from build123d import *

# Parameters (mm, degrees)
SKETCH1_W           = 14.393333334
SKETCH1_H           = 14.393333333
BOSS_EXTRUDE1_DEPTH = 16
FILLET1_R           = 1
SKETCH2_R           = 5.926666667
CUT_EXTRUDE1_DEPTH  = 0.2


with BuildPart() as part:
    # Sketch1 → Boss-Extrude1 (new body)
    with BuildSketch(Plane.XY):
        with Locations((-166.361835023, 44.90232352)):
            Rectangle(SKETCH1_W, SKETCH1_H)
    extrude(amount=BOSS_EXTRUDE1_DEPTH)

    # Fillet1
    fillet1_edges = [part.edges().sort_by_distance(p)[0] for p in [
        (-159.165168356, 37.705656853, 8),
        (-173.55850169, 37.705656853, 8),
        (-173.55850169, 52.098990186, 8),
        (-159.165168356, 52.098990186, 8),
    ]]
    fillet(fillet1_edges, radius=FILLET1_R)

    # Sketch2 → Cut-Extrude1 (cut)
    with BuildSketch(Plane.XY.offset(16)):
        with Locations((-166.361835023, 44.902323519)):
            Circle(SKETCH2_R)
    extrude(amount=-CUT_EXTRUDE1_DEPTH, mode=Mode.SUBTRACT)


solid = part.part
Geometry: final body of the model. Coordinates: model frame, mm. Round coordinates to 2 decimals unless told otherwise and drop trailing zeros.
Q1. Pin query (flat end, axial travel): P1, Ø2, axis at x = -166.5, y = 40.5, coming from the +Z side; P2, Ø4, axis at x = -168.5, y = 49, coming from the -Z side. Return the tip coordinate at first contact, or that it passes through.
Q2. Material intervals for L1, parallel to Z at x = -161.5, y = 44.25; L2, parallel to X at y = 38.5, z = 3.25; L3, parallel to Y at x = -173, z = 15.25, sorted ascending.
Q3. Pull-direction query (Y, two-part tool) for faces 1 (the flat face through (-166, 45, 0)), 2 (the flat face through (-166, 45, 15.8)), 3 (the cylindrical face through (-173.273, 38.006, 8.112)), 4 (the cylindrical face through (-159.45, 51.8, 8.11)); classes: released by +Y, released by -Y, zero draft, split by the parting line, or undercut.
Evaluation:
1. P1: stops at z = 15.8
1. P2: stops at z = 0
2. L1: z = 0 to 15.8
2. L2: x = -173.54 to -159.19
2. L3: y = 37.81 to 52
3. face 1: zero draft
3. face 2: undercut
3. face 3: released by -Y
3. face 4: released by +Y
